The listing builds one solid part. Answer for the finished solid, in the listing's coordinates (mm). A direction names the side the tool comes from. Coordinates: 2 decimals unless noted, no trailing zeros. Order: outer loops, then holes, each group sorted by start corner. A loop starts at its lowest first (then second) coordinate and runs counter-clockwise, first axis right, second up. Notation, with made-up numbers: (-19, 24) - (35, 24) arc R12 ccw to (35, 30) - close; hole circle Ø1 at (16.5, 39.25). An arc over 180 degrees is marked (long way). Use one line per item in the form item = value. Start each with the question number.
Item 1: Section C-C, the plane y = -11 is taken. Write down the section's boundary in (x, z), and give its area (3 significant figures).
Item 2: Section D-D, the plane z = 3.25 is taken. Count the separate pieces of the cut face and the enclosed holes in it, and give its area (3 significant figures).
Item 3: A tool of negligible diameter and unlimited length cuts with its end or side. For faces 4 (the cylindrical face through (-14.248, 16.586, 2.028)), 5 (the cylindrical face through (8.94, 24.18, 2.03)), from which of +Z, -Z, +X, -X, +Y, -Y can it reach the whole face along a straight path? Write none if from no direction.
Item 4: Each of these flat-tipped pins is pushed along its axis until it touches: pin 1 Ø2 at (x, y) = (0, 7) entering from +Z; pin 2 Ø1.5 at (x, y) = (0, -11) entering from -Z; pin 3 Ø2 at (y, z) = (20.5, 2) entering from +X; pin 4 Ø1.5 at (x, z) = (7.5, 2) entering from -Y. Where does it stop, or does it pass through?
Item 5: Section A-A, the plane y = 0 is taken. Write down the section's boundary in (x, z).
Item 6: Section B-B, the plane x = 0 is taken. Write down the section's boundary in (y, z).
Item 7: The mould has two halves that part along X. Classify faces 1 (the flat face through (14, 20, 2)), 2 (the cylindrical face through (-0.163, 6.268, 2.028)), 3 (the flat face through (-14, 20, 2)): released by +X, released by -X, zero draft, split by the parting line, or undercut.
Item 8: Consider line 1 along X through (y, z) = (-1.5, 1.95); line 2 along Y through (x, z) = (11, 3.15); line 3 along X through (y, z) = (-5, 2.85). Determine where each line is inside the solid, lowest interval first. Write a range as [from, to].
from build123d import *

# Parameters (mm, degrees)
SKETCH1_R         = 21.6
EXTRUDE1_DEPTH    = 4
EXTRUDE2_START    = -4
SKETCH2_R         = 1.25
EXTRUDE2_DEPTH    = 4
FILLET1_R         = 3
FILLET2_R         = 1.5
SKETCH3_R         = 5.5
EXTRUDE3_DEPTH    = 4
SKETCH4_R         = 0.75
EXTRUDE4_DEPTH    = 4
CIRPATTERN1_COUNT = 3
SKETCH5_R         = 1.25
EXTRUDE5_DEPTH    = 4
CIRPATTERN2_COUNT = 3


with BuildPart() as part:
    # Sketch1 → Extrude1 (new body)
    with BuildSketch(Plane.XY):
        Circle(SKETCH1_R)
    extrude(amount=EXTRUDE1_DEPTH)

    # Sketch2 → Extrude2 (add)
    # profile 1 of 2: a face of its own
    with BuildSketch(Plane.XY.offset(4).offset(EXTRUDE2_START)):
        with BuildLine():
            Line((8, 25), (8, 20.063897926))
            ThreePointArc((8, 20.063897926), (11.147528841, 18.501151335), (14, 16.448708156))
            Line((14, 16.448708156), (14, 25))
            Line((14, 25), (8, 25))
        make_face()
        with Locations((11, 22)):
            Circle(SKETCH2_R, mode=Mode.SUBTRACT)
    # profile 2 of 2: a face of its own
    with BuildSketch(Plane.XY.offset(4).offset(EXTRUDE2_START)):
        with BuildLine():
            Line((-14, 25), (-14, 16.448708156))
            ThreePointArc((-14, 16.448708156), (-11.147528841, 18.501151335), (-8, 20.063897926))
            Line((-8, 20.063897926), (-8, 25))
            Line((-8, 25), (-14, 25))
        make_face()
        with Locations((-11, 22)):
            Circle(SKETCH2_R, mode=Mode.SUBTRACT)
    extrude(amount=EXTRUDE2_DEPTH)

    # Fillet1
    fillet1_edges = [part.edges().sort_by_distance(p)[0] for p in [
        (14, 16.448708156, 2),
        (-14, 16.448708156, 2),
        (14, 25, 2),
        (8, 25, 2),
        (-8, 25, 2),
        (-14, 25, 2),
    ]]
    fillet(fillet1_edges, radius=FILLET1_R - 0.0001)  # a hair under: the kernel refuses the full size

    # Fillet2
    fillet2_edges = [part.edges().sort_by_distance(p)[0] for p in [
        (8, 20.063897926, 2),
        (-8, 20.063897926, 2),
    ]]
    fillet(fillet2_edges, radius=FILLET2_R)

    # Sketch3 → Extrude3 (cut)
    with BuildSketch(Plane.XY.offset(4)):
        Circle(SKETCH3_R)
    extrude(amount=-EXTRUDE3_DEPTH, mode=Mode.SUBTRACT)

    # Sketch4 → Extrude4 (cut)
    with BuildSketch(Plane.XY.offset(4)):
        with Locations((0, 7)):
            Circle(SKETCH4_R)
    extrude4 = extrude(amount=-EXTRUDE4_DEPTH, mode=Mode.SUBTRACT)

    # CirPattern1: Extrude4 ×3 about axis
    cirpattern1_axis = Axis((0, 0, 0), (0, 0, 1))
    for i in range(1, CIRPATTERN1_COUNT):
        add(extrude4.rotate(cirpattern1_axis, i * 360 / CIRPATTERN1_COUNT), mode=Mode.SUBTRACT)

    # Sketch5 → Extrude5 (cut)
    with BuildSketch(Plane.XY.offset(4)):
        with Locations((0, -11)):
            Circle(SKETCH5_R)
    extrude5 = extrude(amount=-EXTRUDE5_DEPTH, mode=Mode.SUBTRACT)

    # CirPattern2: Extrude5 ×3 about axis
    cirpattern2_axis = Axis((0, 0, 0), (0, 0, 1))
    for i in range(1, CIRPATTERN2_COUNT):
        add(extrude5.rotate(cirpattern2_axis, i * 360 / CIRPATTERN2_COUNT), mode=Mode.SUBTRACT)


solid = part.part
Response:
q1.outline = (-18.59, 0) - (-1.25, 0) - (-1.25, 4) - (-18.59, 4) - close; (1.25, 0) - (18.59, 0) - (18.59, 4) - (1.25, 4) - close
q1.area = 139 mm2
q2.separate_pieces = 1
q2.enclosed_holes = 9
q2.area = 1,410 mm2
q3.face_4 = +Z, -Z, -X, +Y
q3.face_5 = +Z, -Z, +Y
q4.pin_1 = 4
q4.pin_2 = through
q4.pin_3 = 14
q4.pin_4 = -20.52
q5.outline = (-21.6, 0) - (-5.5, 0) - (-5.5, 4) - (-21.6, 4) - close; (5.5, 0) - (21.6, 0) - (21.6, 4) - (5.5, 4) - close
q6.outline = (-21.6, 0) - (-12.25, 0) - (-12.25, 4) - (-21.6, 4) - close; (-9.75, 0) - (-5.5, 0) - (-5.5, 4) - (-9.75, 4) - close; (5.5, 0) - (6.25, 0) - (6.25, 4) - (5.5, 4) - close; (7.75, 0) - (21.6, 0) - (21.6, 4) - (7.75, 4) - close
q7.face_1 = released by +X
q7.face_2 = undercut
q7.face_3 = released by -X
q8.line_1 = [-21.55, -5.29], [5.29, 21.55]
q8.line_2 = [-18.59, 20.75], [23.25, 25]
q8.line_3 = [-21.01, -2.29], [2.29, 21.01]
